The drawing under review shows one solid part. Ordinate dimensions are in mm from its lowest x, y, z. Give positions to 0.01 mm unless a question says otherwise; leave off trailing zeros. Order: outer loops, then holes, each group sorted by start corner. A loop starts at its lowest first (then second) coordinate and runs counter-clockwise, first axis right, second up. Notation, with made-up numbers: (-6, -6.75) - (45, -6.75) arc R9 cw to (45, 0.25) - close; hole circle Ø7 at (-7.5, 40.25). An arc over 180 degrees is marked (long way). Write item = value, one per line. Start each with the question number.
1. We need section C-C, the plane x = 36.5. Give the boundary of the cut face in (y, z).
2. We need section B-B, the plane x = 335. Give the boundary of the cut face in (y, z).
3. Wall thickness on probe 1 along Y at (x, z) = (335, 2.8): over which ranges is the line inside the solid? List them lowest first.
4. For P1, Ø15, axis at x = 35, y = 17.5, coming from the +Z side, flat-tipped, find the tip position at first contact; note if it passes through.
5. We need section A-A, the plane y = 17.5. Give the boundary of the cut face in (x, z), and give its area (3 significant figures).
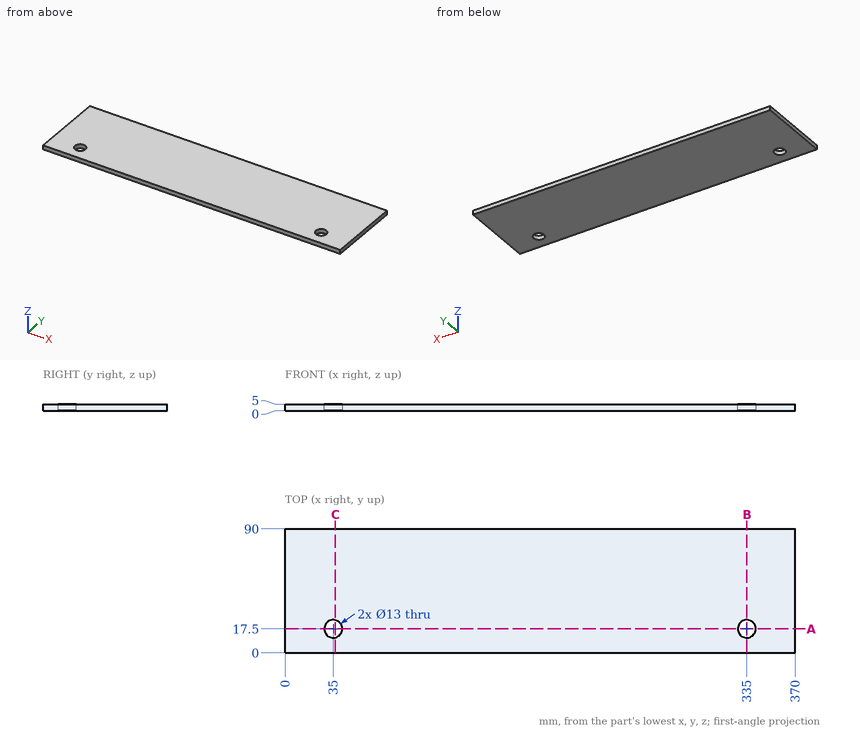
Model answer:
q1.outline = (0, 0) - (11.18, 0) - (11.18, 5) - (0, 5) - close; (23.82, 0) - (90, 0) - (90, 5) - (23.82, 5) - close
q2.outline = (0, 0) - (11, 0) - (11, 5) - (0, 5) - close; (24, 0) - (90, 0) - (90, 5) - (24, 5) - close
q3.probe_1 = 0 to 11, 24 to 90
q4.P1 = 5
q5.outline = (0, 0) - (28.5, 0) - (28.5, 5) - (0, 5) - close; (41.5, 0) - (328.5, 0) - (328.5, 5) - (41.5, 5) - close; (341.5, 0) - (370, 0) - (370, 5) - (341.5, 5) - close
q5.area = 1,720 mm2
